Input: part model. Units: mm. Frame: model coordinates. A direction names the side the tool comes from. Coordinates: 2 decimals unless noted, no trailing zeros. Write each loop counter-clockwise with the first axis right and the second up, starting at its lowest first coordinate (ties: lowest second). Pieces come first, ordered by that corner, then holes. Notation, with made-up numbers: M -36.75,57.5 L -24.75,57.5 A36 cw -24.75,91.5 Z; hole C -7,-4 d8. An arc over 180 degrees is marked long. Use CSV: the item, a comma, the result in double quotes.
```python
from build123d import *

# Parameters (mm, degrees)
SKETCH2_R                       = 12.446
BOSS_EXTRUDE1_DEPTH             = 28.194
CHAMFER1_SIZE                   = 0.508
F_45_0_082_DIAMETER_HOLE1_D     = 2.0828
F_45_0_082_DIAMETER_HOLE1_DEPTH = 21.59
F_45_0_082_DIAMETER_HOLE1_TIP   = 0.431362004
SKETCH11_W                      = 20
SKETCH11_H                      = 20
CUT_EXTRUDE1_DEPTH              = 0.762
CUT_EXTRUDE2_REACH              = 35.237
SKETCH13_W                      = 22.592421824
SKETCH13_H                      = 4.7752
CUT_EXTRUDE3_REACH              = 35.237
SKETCH14_W                      = 4.7752
SKETCH14_H                      = 22.592421824
CIRPATTERN2_COUNT               = 6
SKETCH18_W                      = 0.762
SKETCH18_H                      = 0.508


with BuildPart() as part:
    # Sketch2 → Boss-Extrude1 (new body)
    with BuildSketch(Plane.XY):
        Circle(SKETCH2_R)
    extrude(amount=BOSS_EXTRUDE1_DEPTH)

    # Chamfer1
    chamfer1_edges = [part.edges().sort_by_distance(p)[0] for p in [
        (-12.446, 0, 0),
        (-12.446, 0, 28.194),
    ]]
    chamfer(chamfer1_edges, length=CHAMFER1_SIZE)

    # #45 (0.082) Diameter Hole1
    with Locations(Plane(origin=(0, 0, 0), x_dir=(-1, 0, 0), z_dir=(0, 0, -1))):
        with Locations((0, 8.255), (-7.149039708, 4.1275), (-7.149039708, -4.1275), (0, -8.255), (7.149039708, -4.1275), (7.149039708, 4.1275)):
            Hole(F_45_0_082_DIAMETER_HOLE1_D / 2, depth=F_45_0_082_DIAMETER_HOLE1_DEPTH)
            with Locations((0, 0, -(F_45_0_082_DIAMETER_HOLE1_DEPTH + F_45_0_082_DIAMETER_HOLE1_TIP / 2))):  # 135° drill point
                Cone(0, F_45_0_082_DIAMETER_HOLE1_D / 2, F_45_0_082_DIAMETER_HOLE1_TIP, mode=Mode.SUBTRACT)

    # Sketch11 → Cut-Extrude1 (cut)
    with BuildSketch(Plane.XY.offset(28.194)):
        Rectangle(SKETCH11_W, SKETCH11_H)
    extrude(amount=-CUT_EXTRUDE1_DEPTH, mode=Mode.SUBTRACT)

    # Cut-Extrude2: up to this face of the body (flat: up to its plane)
    cut_extrude2_end = Plane(part.part.faces().sort_by_distance((0, 0, 27.432))[0])
    # Sketch13 → Cut-Extrude2 (cut, up to the picked face)
    with BuildSketch(Plane.XY.offset(28.194), mode=Mode.PRIVATE) as cut_extrude2_sk1:
        with Locations((0, 7.6124)):
            Rectangle(SKETCH13_W, SKETCH13_H)
    cut_extrude2_tool1 = split(extrude(cut_extrude2_sk1.sketch, amount=-CUT_EXTRUDE2_REACH, mode=Mode.PRIVATE), bisect_by=cut_extrude2_end, keep=Keep.BOTH, mode=Mode.PRIVATE)
    # Sketch13 → Cut-Extrude2 (cut, up to the picked face)
    with BuildSketch(Plane.XY.offset(28.194), mode=Mode.PRIVATE) as cut_extrude2_sk2:
        with Locations((0, -7.6124)):
            Rectangle(SKETCH13_W, SKETCH13_H)
    cut_extrude2_tool2 = split(extrude(cut_extrude2_sk2.sketch, amount=-CUT_EXTRUDE2_REACH, mode=Mode.PRIVATE), bisect_by=cut_extrude2_end, keep=Keep.BOTH, mode=Mode.PRIVATE)
    add(cut_extrude2_tool1.solids().sort_by(Axis((0, 7.6124, 28.194), (0, 0, -1)))[0], mode=Mode.SUBTRACT)
    add(cut_extrude2_tool2.solids().sort_by(Axis((0, -7.6124, 28.194), (0, 0, -1)))[0], mode=Mode.SUBTRACT)

    # Cut-Extrude3: up to this face of the body (flat: up to its plane)
    cut_extrude3_end = Plane(part.part.faces().sort_by_distance((0, 0, 27.432))[0])
    # Sketch14 → Cut-Extrude3 (cut, up to the picked face)
    with BuildSketch(Plane.XY.offset(28.194), mode=Mode.PRIVATE) as cut_extrude3_sk1:
        with Locations((-7.6124, 0)):
            Rectangle(SKETCH14_W, SKETCH14_H)
    cut_extrude3_tool1 = split(extrude(cut_extrude3_sk1.sketch, amount=-CUT_EXTRUDE3_REACH, mode=Mode.PRIVATE), bisect_by=cut_extrude3_end, keep=Keep.BOTH, mode=Mode.PRIVATE)
    # Sketch14 → Cut-Extrude3 (cut, up to the picked face)
    with BuildSketch(Plane.XY.offset(28.194), mode=Mode.PRIVATE) as cut_extrude3_sk2:
        with Locations((7.6124, 0)):
            Rectangle(SKETCH14_W, SKETCH14_H)
    cut_extrude3_tool2 = split(extrude(cut_extrude3_sk2.sketch, amount=-CUT_EXTRUDE3_REACH, mode=Mode.PRIVATE), bisect_by=cut_extrude3_end, keep=Keep.BOTH, mode=Mode.PRIVATE)
    add(cut_extrude3_tool1.solids().sort_by(Axis((-7.6124, 0, 28.194), (0, 0, -1)))[0], mode=Mode.SUBTRACT)
    add(cut_extrude3_tool2.solids().sort_by(Axis((7.6124, 0, 28.194), (0, 0, -1)))[0], mode=Mode.SUBTRACT)

    # Sketch17 → Cut-Revolve2 (revolve, cut)
    with BuildSketch(Plane(origin=(0, 0, 0), x_dir=(0, 0, -1), z_dir=(1, 0, 0)), mode=Mode.PRIVATE) as cut_revolve2_sk:
        Polygon((-20.510254982, 8.255), (-20.510254982, 9.271), (-7.62, 11.255), (0, 11.255), (0, 8.255), (-7.62, 8.255), align=None)
    cut_revolve2 = revolve(cut_revolve2_sk.sketch.rotate(Axis((0, 8.255, 20.510254982), (0, 0, -1)), 270), axis=Axis((0, 8.255, 20.510254982), (0, 0, -1)), mode=Mode.SUBTRACT)

    # CirPattern2: Cut-Revolve2 ×6 about axis
    cirpattern2_axis = Axis((0, 0, 0), (0, 0, 1))
    for i in range(1, CIRPATTERN2_COUNT):
        add(cut_revolve2.rotate(cirpattern2_axis, i * 360 / CIRPATTERN2_COUNT), mode=Mode.SUBTRACT)

    # Sketch18 → Cut-Revolve3 (revolve, cut)
    with BuildSketch(Plane(origin=(0, 0, 0), x_dir=(0, 0, -1), z_dir=(1, 0, 0)), mode=Mode.PRIVATE) as cut_revolve3_sk:
        with Locations((-1.651, 12.192)):
            Rectangle(SKETCH18_W, SKETCH18_H)
    revolve(cut_revolve3_sk.sketch.rotate(Axis((0, 0, 27.686), (0, 0, -1)), 90), axis=Axis((0, 0, 27.686), (0, 0, -1)), mode=Mode.SUBTRACT)


solid = part.part
```
1. Access query for faces 1 (the cylindrical face through (-2.588, 11.654, 1.646)), 2 (the conical face through (-12.075, 0.077, 28.056)), 3 (the cylindrical face through (8.1, 3.7, 21)). Directions: +Z, -Z, +X, -X, +Y, -Y. A direction counts if a zero-diameter tool reaches every point of the face in a straight line with its end or side. Return the directions, or none.
Resolved:
face 1,"none"
face 2,"+Z, -X"
face 3,"-Z"
2. Mould query, pull axis Y, two halves, no side actions, for faces 4 (the conical face through (7.1, 4.1, 22)), 5 (the conical face through (0.077, 12.075, 28.056)), 6 (the conical face through (12.075, -0.077, 28.056)). Classes: pulls with the +Y half, pulls with the -Y half, needs draft (parallel to the pull), parting line crosses it, or undercut.
Resolved:
face 4,"undercut"
face 5,"pulls with the +Y half"
face 6,"parting line crosses it"
3. Contact query for flat-ended pins moving along their axis: pin 1 Ø3.5 at (x, y) = (-7.15, -4.13) entering from +Z; pin 2 Ø8 at (x, z) = (8, 23.5) entering from +Y; pin 3 Ø0.8 at (x, z) = (-10.5, 28) entering from +Y. Output: stop coordinate, or through.
Resolved:
pin 1,"stops at z = 27.43"
pin 2,"stops at y = 11.79"
pin 3,"stops at y = 5.22"
4. Material intervals for line 1 (Y direction, x = 0, z = 5.25) (3 decimals); line 2 (Y direction, x = 0, z = 21); line 3 (X direction, y = 4.5, z = 7.5), sorted ascending. Write a range as [from, to].
Resolved:
line 1,"y = [-12.446, -11.255], [-5.255, 5.255], [11.255, 12.446]"
line 2,"y = [-12.45, -9.3], [-7.21, 7.21], [9.3, 12.45]"
line 3,"x = [-11.6, -10.13], [-4.17, 4.17], [10.13, 11.6]"
5. Section C-C (z = 24.75). Return loops of the section in (x, y).
Resolved:
outline,"C 0,0 d24.89"
6. Section A-A (z = 17.75). Return loops of the section in (x, y) (1 decimal), then the cut area to 3 significant figures.
Resolved:
outline,"C 0,0 d24.9; hole C -7.1,-4.1 d2.9; hole C -7.1,4.1 d2.9; hole C 0,-8.3 d2.9; hole C 0,8.3 d2.9; hole C 7.1,-4.1 d2.9; hole C 7.1,4.1 d2.9"
area,"448 mm^2"
7. Section B-B (y = 0). Return loops of the section in (x, z).
Resolved:
outline,"M -12.45,0.51 L -11.94,0 L 11.94,0 L 12.45,0.51 L 12.45,1.27 L 11.94,1.27 L 11.94,2.03 L 12.45,2.03 L 12.45,27.69 L 11.94,28.19 L 10,28.19 L 10,27.43 L -10,27.43 L -10,28.19 L -11.94,28.19 L -12.45,27.69 L -12.45,2.03 L -11.94,2.03 L -11.94,1.27 L -12.45,1.27 Z"
